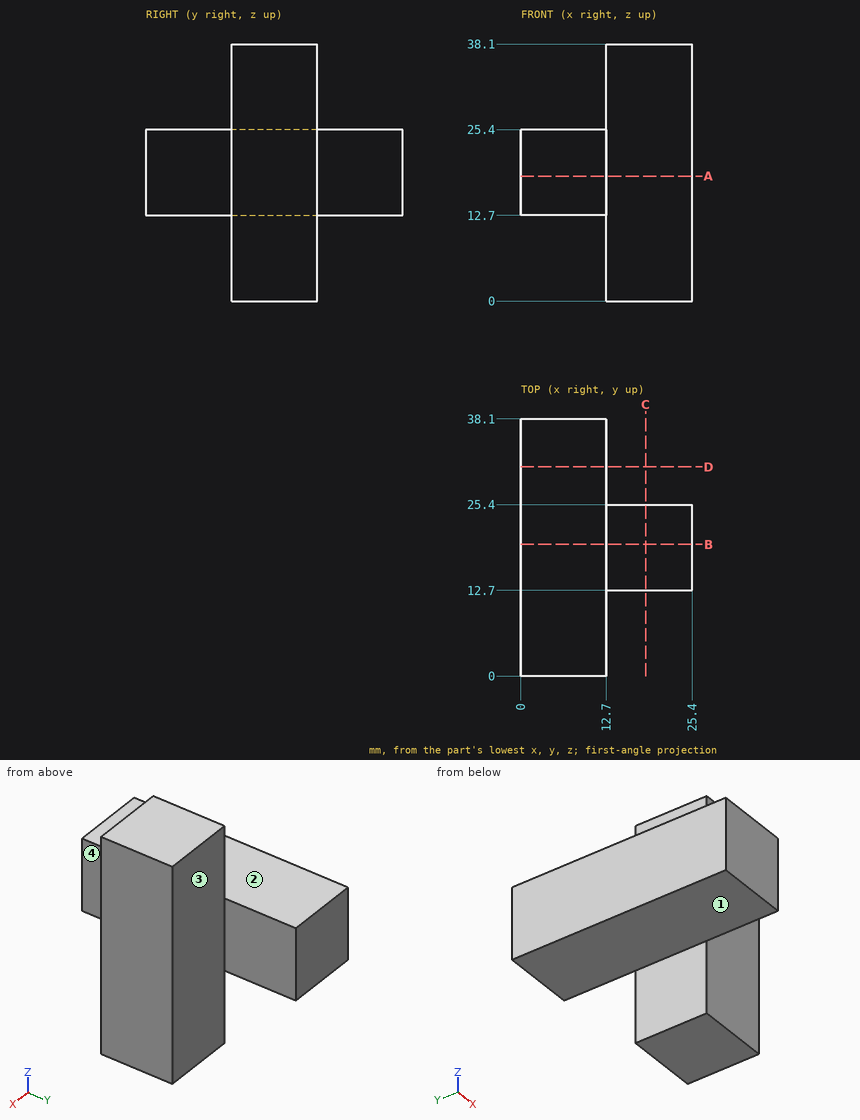
Here's the drawing with two shaded views (mm, measured from the low corner). I have some questions. A direction names the side the tool comes from. Give positions to 0.01 mm unless a question says otherwise; leave off trailing zeros. Order: outer loops, then holes, each group sorted by start corner. A loop starts at its lowest first (then second) coordinate and runs counter-clockwise, first axis right, second up. Notation, with made-up numbers: M 8.5,-40 L 34.5,-40 A26 cw 34.5,-12 Z; hole C -1,18.25 d5. An arc over 180 degrees is marked long. Answer as a JSON object with one key per item and string values. Group by question number.
1) On a 3-axis mill with a long thin cutter (end or side, diameter ignored), from which of +Z, -Z, +X, -X, +Y, -Y can I reach the whole of each face in a straight line? I mean the marked faces 1, 2, 3 and 4. Say none if no direction works.
2) Please list where this line runs through material, in increasing order: L1, parallel to Z at x = 7, y = 17. Write a range as [from, to].
3) Suppose I cut it at C-C, the plane x = 18.5. Write out the boundary of the cut face in (y, z).
4) Suppose I cut it at A-A, the plane z = 18.5. Write out the boundary of the cut face in (x, y), plus the area to 3 significant figures.
5) Suppose I cut it at B-B, the plane y = 19.5. Write out the boundary of the cut face in (x, z).
6) I'm going to push flat-ended pins straight in: pin 1 Ø14 at (x, z) = (22, 14.5) entering from -Y; pin 2 Ø4 at (x, y) = (5.5, 18.5) entering from +Z; pin 3 Ø6.5 at (y, z) = (16, 32) entering from -X. Where does each tip first touch, or does it pass through?
7) Suppose I cut it at D-D, the plane y = 31. Write out the boundary of the cut face in (x, z), plus the area to 3 significant figures.
Results found:
{
 "1": {"face 1": "-Z, -X, +Y, -Y", "face 2": "+Z, -X, +Y, -Y", "face 3": "+Z, -Z, +X, +Y", "face 4": "+Z, -Z, +X, -Y"},
 "2": {"L1": "[12.7, 25.4]"},
 "3": {"outline": "M 12.7,0 L 25.4,0 L 25.4,38.1 L 12.7,38.1 Z"},
 "4": {"outline": "M 0,0 L 12.7,0 L 12.7,12.7 L 25.4,12.7 L 25.4,25.4 L 12.7,25.4 L 12.7,38.1 L 0,38.1 Z", "area": "645 mm²"},
 "5": {"outline": "M 0,12.7 L 12.7,12.7 L 12.7,0 L 25.4,0 L 25.4,38.1 L 12.7,38.1 L 12.7,25.4 L 0,25.4 Z"},
 "6": {"pin 1": "y = 12.7", "pin 2": "z = 25.4", "pin 3": "x = 12.7"},
 "7": {"outline": "M 0,12.7 L 12.7,12.7 L 12.7,25.4 L 0,25.4 Z", "area": "161 mm²"}
}
